The figure shows three views and two pictorial views of one solid part (mm, origin at its lowest corner). Answer the questions. Round coordinates to 2 decimals unless told otherwise and drop trailing zeros. Loops run counter-clockwise (first coordinate to the right, second up) from the corner with the lowest first, then second, coordinate; pieces in that order, holes last. Notation, with made-up numbers: (46.5, -7) -> (85.5, -7) arc R16 ccw to (85.5, 5) -> close; hole circle Ø4 at (18, 85.5). An arc over 180 degrees is marked (long way). Put each result on its own line as item: value.
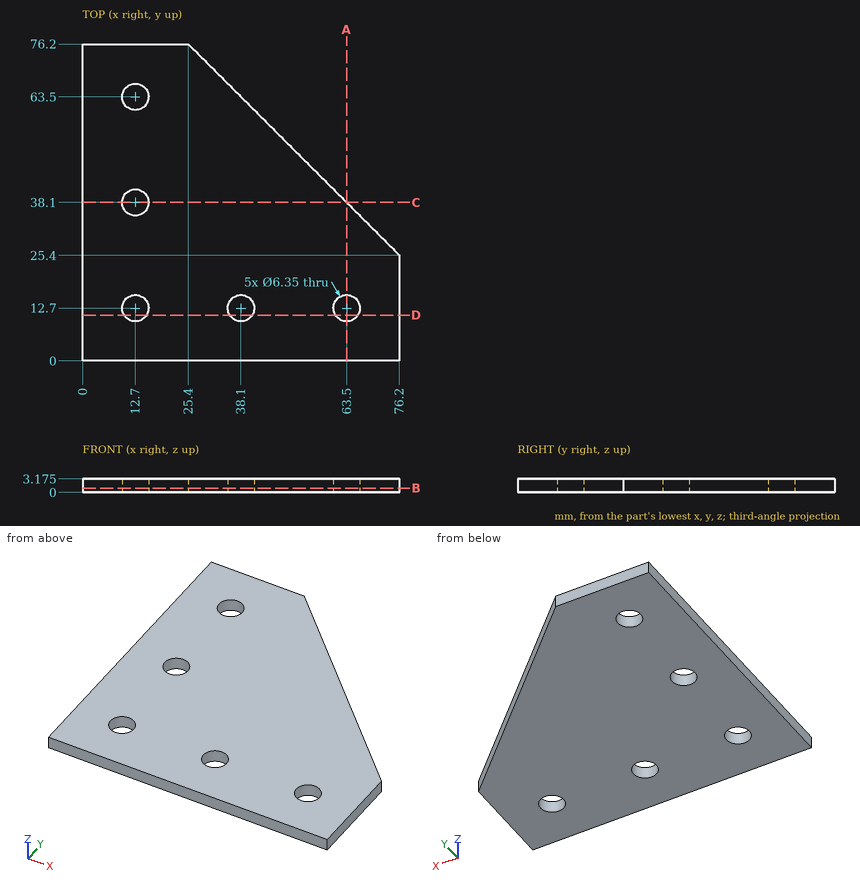
Item 1: The part is cut by section D-D (y = 11). Determine the outline of the cut face in (x, z) (3 decimals), then the cut area to 3 significant figures.
Derived:
outline: (0, 0) -> (10.018, 0) -> (10.018, 3.175) -> (0, 3.175) -> close; (15.382, 0) -> (35.418, 0) -> (35.418, 3.175) -> (15.382, 3.175) -> close; (40.782, 0) -> (60.818, 0) -> (60.818, 3.175) -> (40.782, 3.175) -> close; (66.182, 0) -> (76.2, 0) -> (76.2, 3.175) -> (66.182, 3.175) -> close
area: 191 mm^2
Item 2: The part is cut by section B-B (z = 1). Determine the outline of the cut face in (x, y) (3 decimals), then the cut area to 3 significant figures.
Derived:
outline: (0, 0) -> (76.2, 0) -> (76.2, 25.4) -> (25.4, 76.2) -> (0, 76.2) -> close; hole circle Ø6.35 at (12.7, 12.7); hole circle Ø6.35 at (12.7, 38.1); hole circle Ø6.35 at (12.7, 63.5); hole circle Ø6.35 at (38.1, 12.7); hole circle Ø6.35 at (63.5, 12.7)
area: 4,360 mm^2
Item 3: Find the intervals of material crossed by line 1 along Y through (x, z) = (12.7, 2.2) (3 decimals); line 2 along Y through (x, z) = (11.5, 0.3), in increasing order.
Derived:
line 1: y = 0 to 9.525, 15.875 to 34.925, 41.275 to 60.325, 66.675 to 76.2
line 2: y = 0 to 9.76, 15.64 to 35.16, 41.04 to 60.56, 66.44 to 76.2
Item 4: The part is cut by section A-A (x = 63.5). Determine the outline of the cut face in (y, z) (3 decimals).
Derived:
outline: (0, 0) -> (9.525, 0) -> (9.525, 3.175) -> (0, 3.175) -> close; (15.875, 0) -> (38.1, 0) -> (38.1, 3.175) -> (15.875, 3.175) -> close
Item 5: Flat-ended cylindrical pins translate along their axes: pin 1 Ø5 at (x, y) = (63.5, 12.7) entering from +Z; pin 2 Ø1 at (y, z) = (49, 0.5) entering from +X. Find the tip coordinate at first contact, or state that the pin passes through.
Derived:
pin 1: passes through
pin 2: stops at x = 53.1
Item 6: The part is cut by section C-C (y = 38.1). Determine the outline of the cut face in (x, z) (3 decimals).
Derived:
outline: (0, 0) -> (9.525, 0) -> (9.525, 3.175) -> (0, 3.175) -> close; (15.875, 0) -> (63.5, 0) -> (63.5, 3.175) -> (15.875, 3.175) -> close
